The listing builds one solid part. Answer for the finished solid, in the listing's coordinates (mm). A direction names the side the tool comes from. Round coordinates to 2 decimals unless told otherwise and drop trailing zeros. Write each loop counter-clockwise with the first axis right and the second up, starting at its lowest first coordinate (ties: lowest second). Pieces come first, ordered by that corner, then holes. Notation, with made-up numbers: (67, 71.25) - (100, 71.25) arc R20 ccw to (100, 76.25) - close; hole circle Ø3 at (89.5, -4.75). An arc over 180 degrees is marked (long way). Return JSON: item names as keys, results as strings. Group by question number.
(1) Find the intervals of material crossed by line 1 along Z through (x, y) = (31, 175); line 2 along Y through (x, z) = (5.5, -40.5); line 3 along Y through (x, z) = (49.5, -41), in increasing order. Write a range as [from, to].
(2) Determine the mould class of faces 1 (the flat face through (30, 200, -30)), 2 (the flat face through (8, 194, -29)), 3 (the flat face through (30, 99, -60)) for opening direction Y: +Y half, -Y half, draft (parallel to the pull), parting line (faces both ways), or undercut.
(3) Section B-B, the plane z = -45 is taken. Give the number of separate pieces and of enclosed holes in the cut face, then the cut area to 3 significant figures.
(4) Section A-A, the plane y = 159.72 is taken. Write down the section's boundary in (x, z) (3 decimals).
(5) Each of these flat-tipped pins is pushed along its axis until it touches: pin 1 (8 mm diameter, centred on x = 27.5, y = 26, fed in from +Z); pin 2 (8 mm diameter, centred on x = 17.5, z = -35, fed in from -Y); pin 3 (5 mm diameter, centred on x = 38, y = 171, fed in from +Z). Where does it stop, or does it pass through?
(6) Which of the six approach directions +Z, -Z, +X, -X, +Y, -Y give full straight-line access (tool end or side, diameter ignored) to faces 4 (the cylindrical face through (1.479, 146.855, -34.693)), 5 (the flat face through (44, 125, -56.6)), 6 (the flat face through (52, 5, -29)), 7 (the flat face through (1, 100, 0)), 8 (the flat face through (30, 0, -30))?
(7) Section D-D, the plane z = -8 is taken. Write down the section's boundary in (x, y), then the cut area to 3 significant figures.
(8) Section C-C, the plane x = 44 is taken. Write down the section's boundary in (y, z), then the cut area to 3 significant figures.
```python
from build123d import *

# Parameters (mm, degrees)
SZKIC1_W                    = 60
SZKIC1_H                    = 60
DODANIE_WYCI_GNI_CIE1_DEPTH = 200
SKORUPA1_T                  = -3
SZKIC2_W                    = 5
SZKIC2_H                    = 5
SZKIC2_R                    = 1
DODANIE_WYCI_GNI_CIE5_DEPTH = 57
SZKIC3_W                    = 5
SZKIC3_H                    = 5
SZKIC3_R                    = 1
DODANIE_WYCI_GNI_CIE6_DEPTH = 57
SZKIC4_W                    = 5
SZKIC4_H                    = 5
SZKIC4_R                    = 1
DODANIE_WYCI_GNI_CIE7_DEPTH = 57
SZKIC5_W                    = 5
SZKIC5_H                    = 5
SZKIC5_R                    = 1
DODANIE_WYCI_GNI_CIE8_DEPTH = 57
SZKIC10_R                   = 12.875
WYTNIJ_WYCI_GNI_CIE3_DEPTH  = 3
SZKIC12_W                   = 31.15
SZKIC12_H                   = 7.6
DODANIE_WYCI_GNI_CIE9_DEPTH = 26.5
SZKIC13_R                   = 1.5
WYTNIJ_WYCI_GNI_CIE4_DEPTH  = 5
SZKIC15_R                   = 1.5
WYTNIJ_WYCI_GNI_CIE5_DEPTH  = 5
WYTNIJ_WYCI_GNI_CIE6_DEPTH  = 10
WYTNIJ_WYCI_GNI_CIE7_DEPTH  = 10


with BuildPart() as part:
    # Szkic1 → Dodanie-wyciągnięcie1 (new body)
    with BuildSketch(Plane(origin=(0, 0, 0), x_dir=(1, 0, 0), z_dir=(0, 1, 0))):
        with Locations((30, 30)):
            Rectangle(SZKIC1_W, SZKIC1_H)
    extrude(amount=DODANIE_WYCI_GNI_CIE1_DEPTH)

    # Skorupa1
    skorupa1_openings = [part.faces().sort_by_distance(p)[0] for p in [
        (30, 100, 0),
    ]]
    offset(amount=SKORUPA1_T, openings=skorupa1_openings, kind=Kind.INTERSECTION)

    # Szkic2 → Dodanie-wyciągnięcie5 (add)
    with BuildSketch(Plane.XY.offset(-57)):
        with Locations((5.5, 194.5)):
            Rectangle(SZKIC2_W, SZKIC2_H)
        with Locations(Location((5.5, 194.5, 0), (0, 0, 180))):
            Circle(SZKIC2_R, mode=Mode.SUBTRACT)
    extrude(amount=DODANIE_WYCI_GNI_CIE5_DEPTH)

    # Szkic3 → Dodanie-wyciągnięcie6 (add)
    with BuildSketch(Plane.XY.offset(-57)):
        with Locations((54.5, 194.5)):
            Rectangle(SZKIC3_W, SZKIC3_H)
        with Locations(Location((54.5, 194.5, 0), (0, 0, 180))):
            Circle(SZKIC3_R, mode=Mode.SUBTRACT)
    extrude(amount=DODANIE_WYCI_GNI_CIE6_DEPTH)

    # Szkic4 → Dodanie-wyciągnięcie7 (add)
    with BuildSketch(Plane.XY):
        with Locations((5.5, 5.5)):
            Rectangle(SZKIC4_W, SZKIC4_H)
        with Locations((5.5, 5.5)):
            Circle(SZKIC4_R, mode=Mode.SUBTRACT)
    extrude(amount=-DODANIE_WYCI_GNI_CIE7_DEPTH)

    # Szkic5 → Dodanie-wyciągnięcie8 (add)
    with BuildSketch(Plane.XY.offset(-57)):
        with Locations((54.5, 5.5)):
            Rectangle(SZKIC5_W, SZKIC5_H)
        with Locations(Location((54.5, 5.5, 0), (0, 0, 180))):
            Circle(SZKIC5_R, mode=Mode.SUBTRACT)
    extrude(amount=DODANIE_WYCI_GNI_CIE8_DEPTH)

    # Szkic10 → Wytnij-wyciągnięcie3 (cut)
    with BuildSketch(Plane.ZY):
        with Locations((-34.18, 159.72)):
            Circle(SZKIC10_R)
    extrude(amount=-WYTNIJ_WYCI_GNI_CIE3_DEPTH, mode=Mode.SUBTRACT)

    # Szkic12 → Dodanie-wyciągnięcie9 (add)
    with BuildSketch(Plane.ZY.offset(-57)):
        with Locations((-41.025, 173.56)):
            Rectangle(SZKIC12_W, SZKIC12_H)
        with Locations((-41.025, 124.96)):
            Rectangle(SZKIC12_W, SZKIC12_H)
    extrude(amount=DODANIE_WYCI_GNI_CIE9_DEPTH)

    # Szkic13 → Wytnij-wyciągnięcie4 (cut)
    with BuildSketch(Plane.ZY.offset(-30.5)):
        with Locations((-29.45, 175.36)):
            Circle(SZKIC13_R)
        with Locations((-39.1, 175.36)):
            Circle(SZKIC13_R)
    extrude(amount=-WYTNIJ_WYCI_GNI_CIE4_DEPTH, mode=Mode.SUBTRACT)

    # Szkic15 → Wytnij-wyciągnięcie5 (cut)
    with BuildSketch(Plane.ZY.offset(-30.5)):
        with Locations((-29.45, 124.16)):
            Circle(SZKIC15_R)
        with Locations((-39.1, 124.16)):
            Circle(SZKIC15_R)
    extrude(amount=-WYTNIJ_WYCI_GNI_CIE5_DEPTH, mode=Mode.SUBTRACT)

    # Szkic16 → Wytnij-wyciągnięcie6 (cut)
    with BuildSketch(Plane(origin=(0, 177.36, 0), x_dir=(1, 0, 0), z_dir=(0, 1, 0))):
        Polygon((57, 25.45), (57, 49.45), (47, 25.45), align=None)
    extrude(amount=-WYTNIJ_WYCI_GNI_CIE6_DEPTH, mode=Mode.SUBTRACT)

    # Szkic17 → Wytnij-wyciągnięcie7 (cut)
    with BuildSketch(Plane.ZY):
        with BuildLine():
            Line((-37.93, 172.345), (-37.93, 176.655))
            ThreePointArc((-37.93, 176.655), (-34.18, 180.405), (-30.43, 176.655))
            Line((-30.43, 176.655), (-30.43, 172.345))
            Line((-30.43, 172.345), (-30.43, 171.694400649))
            Line((-30.43, 171.694400649), (-37.93, 171.775211529))
            Line((-37.93, 171.775211529), (-37.93, 172.345))
        make_face()
    extrude(amount=-WYTNIJ_WYCI_GNI_CIE7_DEPTH, mode=Mode.SUBTRACT)


solid = part.part
```
Working result:
{
 "1": {"line 1": "z = [-60, -57], [-56.6, -40.56], [-37.64, -30.91], [-27.99, -25.45]", "line 2": "y = [0, 4.5], [6.5, 8], [192, 193.5], [195.5, 200]", "line 3": "y = [0, 3], [121.16, 128.76], [169.76, 177.36], [197, 200]"},
 "2": {"face 1": "+Y half", "face 2": "undercut", "face 3": "draft"},
 "3": {"separate pieces": "2", "enclosed holes": "4", "area": "1,960 mm^2"},
 "4": {"outline": "(0, -60) - (60, -60) - (60, 0) - (57, 0) - (57, -57) - (3, -57) - (3, -47.055) - (0, -47.055) - close; (0, -21.305) - (3, -21.305) - (3, 0) - (0, 0) - close"},
 "5": {"pin 1": "stops at z = -57", "pin 2": "stops at y = 0", "pin 3": "stops at z = -25.45"},
 "6": {"face 4": "-X", "face 5": "none", "face 6": "+Z", "face 7": "+Z, +X, -X, +Y, -Y", "face 8": "+Z, -Z, +X, -X, -Y"},
 "7": {"outline": "(0, 0) - (60, 0) - (60, 200) - (0, 200) - close; hole (3, 8) - (8, 8) - (8, 3) - (52, 3) - (52, 8) - (57, 8) - (57, 192) - (52, 192) - (52, 197) - (8, 197) - (8, 192) - (3, 192) - close; hole circle Ø2 at (5.5, 5.5); hole circle Ø2 at (5.5, 194.5); hole circle Ø2 at (54.5, 5.5); hole circle Ø2 at (54.5, 194.5)", "area": "1,610 mm^2"},
 "8": {"outline": "(0, -60) - (200, -60) - (200, 0) - (197, 0) - (197, -57) - (3, -57) - (3, 0) - (0, 0) - close; (121.16, -56.6) - (128.76, -56.6) - (128.76, -25.45) - (121.16, -25.45) - close; (169.76, -56.6) - (177.36, -56.6) - (177.36, -25.45) - (169.76, -25.45) - close", "area": "1,420 mm^2"}
}
